from build123d import *

# Parameters (mm, degrees)
BOSS_EXTRUDE1_DEPTH = 6.35
SKETCH17_W          = 196.1896
SKETCH17_H          = 657.6157706
BOSS_EXTRUDE2_DEPTH = 6.35
SKETCH18_W          = 208.8896
SKETCH18_H          = 467.912654328
BOSS_EXTRUDE3_DEPTH = 6.35
SKETCH20_W          = 174.9552
SKETCH20_H          = 101.6
BOSS_EXTRUDE4_DEPTH = 25.4
SKETCH22_W          = 39.8272
SKETCH22_H          = 79.88897833
BOSS_EXTRUDE5_DEPTH = 101.6
SKETCH25_R          = 4.826
CUT_EXTRUDE1_DEPTH  = 6.35


with BuildPart() as part:
    # Sketch15 → Boss-Extrude1 (new body)
    with BuildSketch(Plane(origin=(0, 0, 0), x_dir=(0, 0, -1), z_dir=(1, 0, 0))):
        Polygon((0, 0), (-657.6157706, 0), (-657.6157706, 204.204861602), (-309.033798252, 204.204861602), (-309.033798252, 467.912654328), (0, 467.912654328), align=None)
    boss_extrude1 = extrude(amount=-BOSS_EXTRUDE1_DEPTH)

    # Sketch17 → Boss-Extrude2 (add)
    with BuildSketch(Plane(origin=(0, 0, 0), x_dir=(1, 0, 0), z_dir=(0, 1, 0))):
        with Locations((98.0948, -328.8078853)):
            Rectangle(SKETCH17_W, SKETCH17_H)
    extrude(amount=BOSS_EXTRUDE2_DEPTH)

    # Mirror1: Boss-Extrude1 across plane
    add(boss_extrude1.mirror(Plane(origin=(98.0948, 0, 0), x_dir=(0, 0, 1), z_dir=(1, 0, 0))))

    # Sketch18 → Boss-Extrude3 (add)
    with BuildSketch(Plane(origin=(0, 0, 0), x_dir=(-1, 0, 0), z_dir=(0, 0, -1))):
        with Locations((-98.0948, 233.956327164)):
            Rectangle(SKETCH18_W, SKETCH18_H)
    extrude(amount=-BOSS_EXTRUDE3_DEPTH)

    # Sketch20 → Boss-Extrude4 (add)
    with BuildSketch(Plane(origin=(0, 0, 0), x_dir=(1, 0, 0), z_dir=(0, 1, 0))):
        with Locations((-93.8276, -170.785936787)):
            Rectangle(SKETCH20_W, SKETCH20_H)
        with Locations((290.0172, -170.785936787)):
            Rectangle(SKETCH20_W, SKETCH20_H)
    extrude(amount=BOSS_EXTRUDE4_DEPTH)

    # Sketch22 → Boss-Extrude5 (add)
    with BuildSketch(Plane(origin=(0, 0, 0), x_dir=(1, 0, 0), z_dir=(0, 1, 0))):
        with Locations((-26.2636, -612.31684817)):
            Rectangle(SKETCH22_W, SKETCH22_H)
        with Locations((222.4532, -612.31684817)):
            Rectangle(SKETCH22_W, SKETCH22_H)
    extrude(amount=BOSS_EXTRUDE5_DEPTH)

    # Sketch25 → Cut-Extrude1 (cut)
    with BuildSketch(Plane.ZY.offset(6.35)):
        with Locations((533.1557706, 178.804861602)):
            Circle(SKETCH25_R)
        with Locations((431.5557706, 178.804861602)):
            Circle(SKETCH25_R)
        with Locations((329.9557706, 178.804861602)):
            Circle(SKETCH25_R)
        with Locations((255.439798252, 280.460654328)):
            Circle(SKETCH25_R)
        with Locations((255.439798252, 382.060654328)):
            Circle(SKETCH25_R)
    cut_extrude1 = extrude(amount=-CUT_EXTRUDE1_DEPTH, mode=Mode.SUBTRACT)

    # Mirror2: Cut-Extrude1 across plane
    add(cut_extrude1.mirror(Plane(origin=(98.0948, 0, 0), x_dir=(0, 0, 1), z_dir=(1, 0, 0))), mode=Mode.SUBTRACT)


solid = part.part
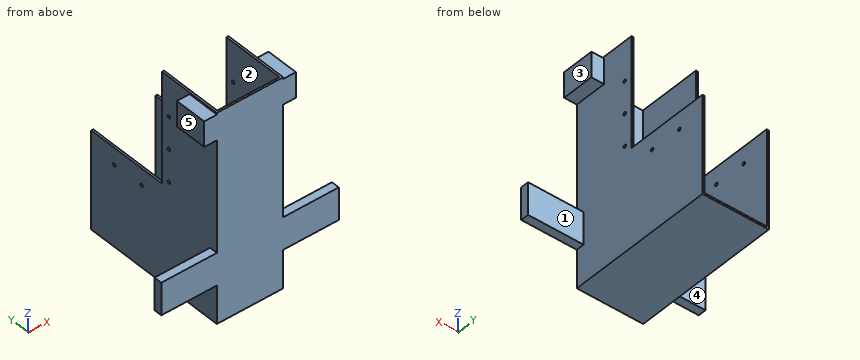
Input: part model. Units: mm. Frame: model coordinates. Face numbers are marked on the shaded views. A direction names the side the tool comes from. Give positions to 0.01 mm unless a question says otherwise; leave off trailing zeros. Write each loop counter-clockwise with the first axis right and the second up, starting at its lowest first coordinate (ties: lowest second). Pieces come first, ordered by that corner, then holes. Notation, with made-up numbers: M 37,9.5 L 91,9.5 A16 ccw 91,15.5 Z; hole C 60,6.5 d8. An arc over 180 degrees is marked long. Use one line per item in the form item = value.
1. Cut plane C-C on x = 90. Return loops of the section in (y, z), and give its area (3 significant figures).
Outcome:
outline = M 0,0 L 467.91,0 L 467.91,6.35 L 6.35,6.35 L 6.35,657.62 L 0,657.62 Z
area = 7,110 mm²
2. Cut plane A-A on z = 487.5. Return loops of the section in (x, y), and give its area (3 significant figures).
Outcome:
outline = M -6.35,0 L 202.54,0 L 202.54,204.2 L 196.19,204.2 L 196.19,6.35 L 0,6.35 L 0,204.2 L -6.35,204.2 Z
area = 3,840 mm²
3. Ray query, L1, parallel to X at y = 142.5, z = 125.5; L2, parallel to Y at x = -71.5, z = 205; L3, parallel to Z at x = 135, y = 82.5. Return the intervals inside material, ascending.
Outcome:
L1 = -6.35 to 0, 196.19 to 202.54
L2 = 0 to 25.4
L3 = 0 to 6.35
4. Cut plane B-B on y = 354.5. Return loops of the section in (x, z).
Outcome:
outline = M -6.35,0 L 202.54,0 L 202.54,309.03 L 196.19,309.03 L 196.19,6.35 L 0,6.35 L 0,309.03 L -6.35,309.03 Z
5. Reachability of the marked faces 1, 2, 3, 4 and 5 from +Z, -Z, +X, -X, +Y, -Y: full face, straight path, thin tool, end or side. Return the list, or none.
Outcome:
face_1 = -Z, +X, +Y
face_2 = +Z, +Y
face_3 = +Z, +X, +Y, -Y
face_4 = -Z, -X, +Y
face_5 = +Z, -X, +Y, -Y
6. Cut plane D-D on z = 159. Return loops of the section in (x, y), and give its area (3 significant figures).
Outcome:
outline = M -181.31,0 L 377.49,0 L 377.49,25.4 L 202.54,25.4 L 202.54,467.91 L 196.19,467.91 L 196.19,6.35 L 0,6.35 L 0,467.91 L -6.35,467.91 L -6.35,25.4 L -181.31,25.4 Z
area = 16,100 mm²
7. First-contact query: P1, Ø12.5, axis at y = 178.8, z = 329.96, coming from the +X side; P2, Ø3, axis at x = -1.5, z = 465.5, coming from the +Y side; P3, Ø24, axis at y = 32.5, z = 625.5, coming from the +X side; P4, Ø2, axis at x = -9, y = 217.5, coming from the -Z side. Flat tips, straight axial feed; report the tip coordinate or a pass-through.
Outcome:
P1 = 202.54
P2 = 204.2
P3 = 242.37
P4 = through
